from build123d import *

# Parameters (mm, degrees)
SKETCH_1_W          = 500.8
SKETCH_1_H          = 300.8
EXTRUDE_1_DEPTH     = 4.75
SKETCH_2_W          = 25.4
SKETCH_2_H          = 25.4
SKETCH_2_W_2        = 4.75
SKETCH_2_H_2        = 80
CUT_EXTRUDE_1_DEPTH = 10
SKETCH_3_R          = 2.150000004
SKETCH_3_R_2        = 2.15
CUT_EXTRUDE_2_DEPTH = 5
SKETCH_4_W          = 80.5
SKETCH_4_H          = 30
CUT_EXTRUDE_3_DEPTH = 4.75
FILLET_1_R          = 7


with BuildPart() as part:
    # 草圖1 → 填料-伸長1 (new body)
    with BuildSketch(Plane.XY):
        Rectangle(SKETCH_1_W, SKETCH_1_H)
    extrude(amount=EXTRUDE_1_DEPTH)

    # 草圖2 → 除料-伸長1 (cut)
    with BuildSketch(Plane(origin=(0, 0, 0), x_dir=(-1, 0, 0), z_dir=(0, 0, -1))):
        with Locations((-237.7, 137.7)):
            Rectangle(SKETCH_2_W, SKETCH_2_H)
        with Locations((-237.7, -137.7)):
            Rectangle(SKETCH_2_W, SKETCH_2_H)
        with Locations((237.7, 137.7)):
            Rectangle(SKETCH_2_W, SKETCH_2_H)
        with Locations((237.7, -137.7)):
            Rectangle(SKETCH_2_W, SKETCH_2_H)
        with Locations((-222.625, 65.4)):
            Rectangle(SKETCH_2_W_2, SKETCH_2_H_2)
        with Locations((-222.625, -65.4)):
            Rectangle(SKETCH_2_W_2, SKETCH_2_H_2)
        with Locations((222.625, 65.4)):
            Rectangle(SKETCH_2_W_2, SKETCH_2_H_2)
        with Locations((222.625, -64.4)):
            Rectangle(SKETCH_2_W_2, SKETCH_2_H_2)
        with Locations((-72.625, 65.4)):
            Rectangle(SKETCH_2_W_2, SKETCH_2_H_2)
        with Locations((77.375, 65.4)):
            Rectangle(SKETCH_2_W_2, SKETCH_2_H_2)
        with Locations((77.375, -65.4)):
            Rectangle(SKETCH_2_W_2, SKETCH_2_H_2)
        with Locations((-72.625, -65.4)):
            Rectangle(SKETCH_2_W_2, SKETCH_2_H_2)
    extrude(amount=-CUT_EXTRUDE_1_DEPTH, mode=Mode.SUBTRACT)

    # 草圖3 → 除料-伸長2 (cut)
    with BuildSketch(Plane.XY.offset(4.75)):
        with Locations((-237.7, 107.300000013)):
            Circle(SKETCH_3_R)
        with Locations((-237.7, 82.800000013)):
            Circle(SKETCH_3_R)
        with Locations((-207.3, 137.700000006)):
            Circle(SKETCH_3_R_2)
        with Locations((-182.8, 137.700000006)):
            Circle(SKETCH_3_R_2)
        with Locations((-237.7, -82.800000001)):
            Circle(SKETCH_3_R_2)
        with Locations((-237.7, -107.300000001)):
            Circle(SKETCH_3_R_2)
        with Locations((237.7, -107.300000007)):
            Circle(SKETCH_3_R)
        with Locations((237.7, -82.800000007)):
            Circle(SKETCH_3_R)
        with Locations((237.7, 107.300000006)):
            Circle(SKETCH_3_R_2)
        with Locations((237.7, 82.800000006)):
            Circle(SKETCH_3_R_2)
        with Locations((182.8, 137.700000006)):
            Circle(SKETCH_3_R_2)
        with Locations((207.3, 137.700000006)):
            Circle(SKETCH_3_R_2)
    extrude(amount=-CUT_EXTRUDE_2_DEPTH, mode=Mode.SUBTRACT)

    # 草圖4 → 除料-伸長3 (cut)
    with BuildSketch(Plane.XY.offset(4.75)):
        with Locations((-2.375, 110.4)):
            Rectangle(SKETCH_4_W, SKETCH_4_H)
    extrude(amount=-CUT_EXTRUDE_3_DEPTH, mode=Mode.SUBTRACT)

    # 圓角1
    fillet_1_edges = [part.edges().sort_by_distance(p)[0] for p in [
        (37.875, 125.4, 2.375),
        (37.875, 95.4, 2.375),
        (-42.625, 95.4, 2.375),
        (-42.625, 125.4, 2.375),
    ]]
    fillet(fillet_1_edges, radius=FILLET_1_R)


solid = part.part
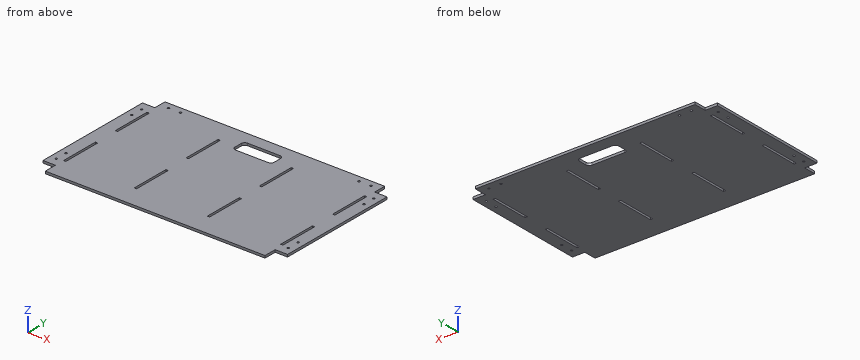
For this review, take the finished solid that the model builds, in its own axes (mm). Round coordinates to 2 decimals unless told otherwise and drop trailing zeros. Order: outer loops, then holes, each group sorted by start corner. A loop starts at its lowest first (then second) coordinate and runs counter-clockwise, first axis right, second up. Notation, with made-up numbers: (69, 64.5) -> (115, 64.5) arc R28 cw to (115, 100.5) -> close; hole circle Ø7 at (37, 70.25). An arc over 180 degrees is marked (long way). Write item = value, one per line. Start each with the question number.
1) Insertion check: pin 1 (4 mm diameter, centred on x = 237.7, y = -82.8, fed in from -Z). The pin has a flat end and moves straight along its axis. Give the tip position at first contact, or say it passes through.
2) Take a section at B-B on y = -93.5. State the section outline as (x, z) points, plus the area to 3 significant figures.
3) To check wall thickness, follow line 1 (X direction, y = -43, z = 1.25); line 2 (Y direction, x = 237.7, z = 2.65); line 3 (Y direction, x = 207.3, z = 2.2). State the ranges of each line that lie inside material, in increasing order. Write a range as from..to.
4) Take a section at C-C on z = 2.9. Count the separate pieces of the cut face and the enclosed holes in it, plus the area to 3 significant figures.
5) Take a section at A-A on x = -15. State the section outline as (y, z) points.
Verdict:
q1.pin_1 = through
q2.outline = (-250.4, 0) -> (-225, 0) -> (-225, 4.75) -> (-250.4, 4.75) -> close; (-220.25, 0) -> (-79.75, 0) -> (-79.75, 4.75) -> (-220.25, 4.75) -> close; (-75, 0) -> (70.25, 0) -> (70.25, 4.75) -> (-75, 4.75) -> close; (75, 0) -> (220.25, 0) -> (220.25, 4.75) -> (75, 4.75) -> close; (225, 0) -> (250.4, 0) -> (250.4, 4.75) -> (225, 4.75) -> close
q2.area = 2,290 mm2
q3.line_1 = -250.4..-225, -220.25..-79.75, -75..70.25, 75..220.25, 225..250.4
q3.line_2 = -125..-109.45, -105.15..-84.95, -80.65..80.65, 84.95..105.15, 109.45..125
q3.line_3 = -150.4..135.55, 139.85..150.4
q4.separate_pieces = 1
q4.enclosed_holes = 21
q4.area = 142,000 mm2
q5.outline = (-150.4, 0) -> (95.4, 0) -> (95.4, 4.75) -> (-150.4, 4.75) -> close; (125.4, 0) -> (150.4, 0) -> (150.4, 4.75) -> (125.4, 4.75) -> close
